Part model, mm, in its own coordinate system. Give positions to 0.01 mm unless a question says otherwise; leave off trailing zeros. Write each loop counter-clockwise with the first axis right and the second up, starting at its lowest first coordinate (ties: lowest second). Pieces come first, ordered by that corner, then holes. Notation, with made-up numbers: (65, 42) - (85, 42) arc R24 cw to (85, 79) - close; hole circle Ø3 at (-36, 5.25). An arc over 180 degrees is marked (long way). Answer in a Markdown table with one row per item. Add a question column.
1. Probe line 1 along X through (y, z) = (-3, -0.5); line 2 along X through (y, z) = (-8, -5); line 3 along Z through (x, y) = (11.5, -5). List the from-to ranges inside material, lowest first.
2. Band-saw the part on A-A on y = -1. Write the cut outline in (x, z).
3. Drop flat-ended pins along their axis: pin 1 Ø5 at (x, y) = (17.5, -3.5) entering from +Z; pin 2 Ø1.5 at (x, y) = (24.5, -3.5) entering from +Z. Give the stop position or say it passes through.
4. Band-saw the part on C-C on y = -3.5. Write the cut outline in (x, z), plus the area to 3 significant figures.
```python
from build123d import *

# Parameters (mm, degrees)
F1_DEPTH = 10
F2_R     = 4.99999


# Not quite as in the source:
# - a fillet or chamfer is up to 0.001 mm smaller than in the source, because OpenCascade refuses the exact size


with BuildPart() as f1:
    # F0 (on Front) → F1 (new body)
    with BuildSketch(Plane.XZ):
        with BuildLine():
            Line((34, -32), (34, 0))
            ThreePointArc((34, 0), (27.4043260233, -8.6977951997), (17, -12))
            ThreePointArc((17, -12), (6.5956739767, -8.6977951997), (0, 0))
            Line((0, 0), (0, -5))
            Line((0, -5), (0, -32))
            Line((0, -32), (34, -32))
        make_face()
    extrude(amount=F1_DEPTH)

    # F2 (radius 5 in the source; OpenCascade refuses exactly that, so slightly less here)
    f2_edges = [f1.edges().sort_by_distance(p)[0] for p in [
        (17, 0, -32),
        (17, -10, -32),
    ]]
    fillet(f2_edges, radius=F2_R)


solid = f1.part
```
Values:
| question | item | result |
|---|---|---|
| 1 | line 1 | x = 0 to 0.19, 33.81 to 34 |
| 1 | line 2 | x = 0 to 2.73, 31.27 to 34 |
| 1 | line 3 | z = -32 to -11.14 |
| 2 | outline | (0, -30) - (34, -30) - (34, 0) arc R18.04 cw to (0, 0) - close |
| 3 | pin 1 | stops at z = -11.75 |
| 3 | pin 2 | stops at z = -10 |
| 4 | outline | (0, -31.77) - (34, -31.77) - (34, 0) arc R18.04 cw to (0, 0) - close |
| 4 | area | 783 mm² |
